Can you work these out from the model? Positions are in its coordinate system, mm. Face numbers are marked on the shaded views. A direction names the side the tool comes from. Give positions to 0.01 mm unless a question says otherwise; leave off trailing zeros. Write each loop counter-clockwise with the first axis right and the second up, starting at its lowest first coordinate (ties: lowest second). Pieces come first, ordered by that corner, then holes. Notation, with made-up numbers: (29, -23.75) - (71, -23.75) arc R16 ccw to (71, -16.75) - close; hole circle Ø10 at (66.25, -12). An arc over 180 degrees is marked (long way). Return JSON: item names as keys, results as strings. Group by question number.
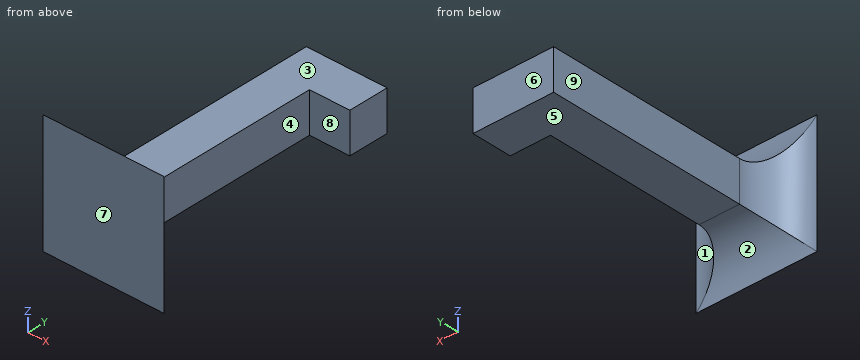
from build123d import *

# Parameters (mm, degrees)
SKETCH1_R           = 5
SKETCH1_R_2         = 10.05
BOSS_EXTRUDE1_DEPTH = 10
SKETCH2_R           = 1.25
CUT_EXTRUDE1_DEPTH  = 10
SKETCH4_R           = 7.5
BOSS_EXTRUDE2_DEPTH = 30
BOSS_EXTRUDE2_TAPER = 7
SKETCH5_R           = 1.25
CUT_EXTRUDE2_DEPTH  = 10
FILLET1_R           = 15
SKETCH6_W           = 5
SKETCH6_H           = 5
BOSS_EXTRUDE3_DEPTH = 30
SKETCH7_W           = 5
SKETCH7_H           = 5
BOSS_EXTRUDE4_DEPTH = 5
FILLET2_R           = 5
SKETCH8_W           = 100
SKETCH8_H           = 10
CUT_EXTRUDE4_DEPTH  = 100


# Some blends are built 0.0001 mm under size
with BuildPart() as part:
    # Sketch1 → Boss-Extrude1 (new body)
    with BuildSketch(Plane(origin=(0, 0, 0), x_dir=(1, 0, 0), z_dir=(0, 1, 0))):
        Polygon((23.995878661, -35), (56.995878661, -35), (56.995878661, -75), (88.995878661, -75), (88.995878661, -25), (88.995878661, 25), (17.5, 25), (-2.004121339, 25), (-2.004121339, 7.840472806), (23.995878661, 7.840472806), (23.995878661, 0), (23.995878661, -28.53803828), (10.495878661, -28.53803828), (10.495878661, -35), align=None)
        with Locations(Location((51.495878661, 0, 0), (0, 0, 270))):
            Circle(SKETCH1_R, mode=Mode.SUBTRACT)
        with Locations(Location((73.995878661, -60, 0), (0, 0, 270))):
            Circle(SKETCH1_R_2, mode=Mode.SUBTRACT)
    extrude(amount=BOSS_EXTRUDE1_DEPTH)

    # Sketch2 → Cut-Extrude1 (cut)
    with BuildSketch(Plane.ZY.offset(-10.495878661)):
        with Locations((31.76901914, 5)):
            Circle(SKETCH2_R)
    extrude(amount=-CUT_EXTRUDE1_DEPTH, mode=Mode.SUBTRACT)

    # Sketch4 → Boss-Extrude2 (add)
    with BuildSketch(Plane(origin=(0, 10, 0), x_dir=(1, 0, 0), z_dir=(0, 1, 0))):
        with Locations((6.495878661, 16.5)):
            Circle(SKETCH4_R)
    extrude(amount=BOSS_EXTRUDE2_DEPTH, taper=BOSS_EXTRUDE2_TAPER)

    # Sketch5 → Cut-Extrude2 (cut)
    with BuildSketch(Plane(origin=(0, 40, 0), x_dir=(1, 0, 0), z_dir=(0, 1, 0))):
        with Locations(Location((6.495878661, 16.5, 0), (0, 0, 270))):
            Circle(SKETCH5_R)
    extrude(amount=-CUT_EXTRUDE2_DEPTH, mode=Mode.SUBTRACT)

    # Fillet1
    # the kernel refuses this fillet: 15 mm, written as the material it adds along each edge
    with BuildSketch(Plane(origin=(56.995878661, 0, 35), x_dir=(-1, 0, 0), z_dir=(0, 1, 0)), Plane(origin=(23.995878661, 0, -7.840472806), x_dir=(-1, 0, 0), z_dir=(0, 1, 0))) as fillet1_piece_1:
        with BuildLine():
            CenterArc((FILLET1_R, FILLET1_R), FILLET1_R, 180, 90)
            Line((0, FILLET1_R), (-FILLET1_R * 0.02, FILLET1_R))
            Line((-FILLET1_R * 0.02, FILLET1_R), (-FILLET1_R * 0.02, -FILLET1_R * 0.02))
            Line((-FILLET1_R * 0.02, -FILLET1_R * 0.02), (FILLET1_R, -FILLET1_R * 0.02))
            Line((FILLET1_R, -FILLET1_R * 0.02), (FILLET1_R, 0))
        make_face()
    extrude(amount=10)
    with BuildSketch(Plane(origin=(23.995878661, 0, 28.53803828), x_dir=(0, 0, -1), z_dir=(0, 1, 0))) as fillet1_piece_2:
        with BuildLine():
            CenterArc((14.924811557, 15), FILLET1_R, 185.739170477, 84.260829523)
            Line((0, 13.5), (-0.298496231, 13.47))
            ThreePointArc((-0.298496231, 13.47), (-0.3, 6.75), (-0.3, 0))
            Line((-0.3, 0), (0, -0.3))
            Line((0, -0.3), (14.924811557, -0.3))
            Line((14.924811557, -0.3), (14.924811557, 0))
        make_face()
    extrude(amount=10)

    # Sketch6 → Boss-Extrude3 (add)
    with BuildSketch(Plane(origin=(0, 10, 0), x_dir=(1, 0, 0), z_dir=(0, 1, 0))):
        with Locations((76.495878661, 17.5)):
            Rectangle(SKETCH6_W, SKETCH6_H)
    extrude(amount=BOSS_EXTRUDE3_DEPTH)

    # Sketch7 → Boss-Extrude4 (add)
    with BuildSketch(Plane(origin=(78.995878661, 0, 0), x_dir=(0, 0, -1), z_dir=(1, 0, 0))):
        with Locations((17.5, 37.5)):
            Rectangle(SKETCH7_W, SKETCH7_H)
    extrude(amount=BOSS_EXTRUDE4_DEPTH)

    # Fillet2
    fillet2_edges = [part.edges().sort_by_distance(p)[0] for p in [
        (78.995878661, 10, -17.5),
        (76.495878661, 10, -20),
        (73.995878661, 10, -17.5),
        (76.495878661, 10, -15),
    ]]
    fillet(fillet2_edges, radius=FILLET2_R - 0.0001)  # a hair under: the kernel refuses the full size

    # Sketch8 → Cut-Extrude4 (cut)
    with BuildSketch(Plane(origin=(88.995878661, 0, 0), x_dir=(0, 0, -1), z_dir=(1, 0, 0))):
        with Locations((-25, 5)):
            Rectangle(SKETCH8_W, SKETCH8_H)
    extrude(amount=-CUT_EXTRUDE4_DEPTH, mode=Mode.SUBTRACT)


with BuildPart() as cut_extrude4_kept_piece:
    # of the separate pieces the step leaves, the one the design keeps (cut_extrude4_pieces_kept)
    add(part.part.solids().sort_by_distance((83.995778661, 10, -24.9999))[0])


solid = cut_extrude4_kept_piece.part
1) Imagine slicing it at C-C, the plane x = 76. Write out the boundary of the cut face in (y, z), and give its area (3 significant figures).
2) We'd pull the mould along Y, two halves only. Please class the marked faces 1, 2, 3 and 4: pulls with the +Y half, pulls with the -Y half, needs draft (parallel to the pull), parting line crosses it, or undercut.
3) Will these pins go through, and if not, where does the flat tip stop? pin 1 Ø4 at (y, z) = (24, -18) entering from +X; pin 2 Ø1.5 at (y, z) = (31.5, -16.5) entering from -X; pin 3 Ø8 at (y, z) = (15, -13) entering from -X.
4) Imagine slicing it at D-D, the plane y = 35.75. Write out the boundary of the cut face in (x, z).
5) I need wall thicknesses on line 1 along Z through (x, y) = (78, 19.25); line 2 along Y through (x, z) = (79.5, -16.25); line 3 along X through (y, z) = (20.75, -17). Which ranges of each line are inside material? Lowest first, please.
6) On a 3-axis mill with a long thin cutter (end or side, diameter ignored), from which of +Z, -Z, +X, -X, +Y, -Y can I reach the whole of each face in a straight line? I mean the marked faces 5, 6, 7, 8 and 9. Say none if no direction works.
7) Imagine slicing it at A-A, the plane x = 82.5. Write out the boundary of the cut face in (y, z), and give its area (3 significant figures).
8) Imagine slicing it at B-B, the plane z = -17.25. Write out the boundary of the cut face in (x, y), and give its area (3 significant figures).
Resolved:
{
 "1": {"outline": "(10, -25) arc R5 cw to (15, -20) - (40, -20) - (40, -15) - (15, -15) arc R5 cw to (10, -10) - close", "area": "161 mm^2"},
 "2": {"face 1": "undercut", "face 2": "pulls with the +Y half", "face 3": "needs draft", "face 4": "undercut"},
 "3": {"pin 1": "x = 79", "pin 2": "x = 74", "pin 3": "x = 72"},
 "4": {"outline": "(74, -20) - (84, -20) - (84, -15) - (74, -15) - close"},
 "5": {"line 1": "-20 to -15", "line 2": "10 to 12.81, 35 to 40", "line 3": "74 to 79"},
 "6": {"face 5": "-Z, +X, -X, +Y", "face 6": "+Z, -Z, +X, -X, +Y", "face 7": "+Z, -Z, +X, -X, -Y", "face 8": "+Z, -Z, +X", "face 9": "+Z, -Z, -X, +Y"},
 "7": {"outline": "(10, -25) arc R5 cw to (10.23, -23.5) - (10.23, -11.5) arc R5 cw to (10, -10) - close; (35, -20) - (40, -20) - (40, -15) - (35, -15) - close", "area": "28.0 mm^2"},
 "8": {"outline": "(69, 10) - (84, 10) arc R5 cw to (79, 15) - (79, 35) - (84, 35) - (84, 40) - (74, 40) - (74, 15) arc R5 cw to start", "area": "186 mm^2"}
}
